Geometry check sheet. Reference: drawing and pictorial views, mm from the part's lowest x, y, z. A direction names the side the tool comes from. Round coordinates to 2 decimals unless told otherwise and drop trailing zeros. Write each loop counter-clockwise with the first axis right and the second up, starting at its lowest first coordinate (ties: lowest second). Pieces come first, ordered by that corner, then holes. Notation, with made-up numbers: M 10,56 L 60,56 A22 cw 60,69 Z; hole C -29.5,51.25 d10. An arc over 180 degrees is marked long. Put each result on its own line as item: value. Start each with the question number.
(1) Section check C-C on y = 46. Record the cut outline in (x, z) (1 decimal).
(2) Gauge pin test, flat ends, axial feed: pin 1 (5 mm diameter, centred on x = 51.5, z = 8, fed in from -Y); pin 2 (12 mm diameter, centred on x = 24, z = 3.5, fed in from +Y); pin 3 (8 mm diameter, centred on x = 60.5, z = 18, fed in from +Y); pin 4 (2.5 mm diameter, centred on x = 20.05, y = 46, fed in from -Z). Record the tip position at first contact, or that the pin passes through.
(3) Section check D-D on x = 26.5. Record the cut outline in (y, z) (1 decimal), then the cut area to 3 significant figures.
(4) Material ranges on probe 1 along Y at (x, z) = (36.5, 1.15); probe 2 along Y at (x, z) = (36, 6) (1 decimal); probe 3 along Y at (x, z) = (37.5, 27.5) (1 decimal), recorded low to high.
(5) Section check B-B on z = 18.5. Record the cut outline in (x, y) (1 decimal).
(6) Mould release check, pull along Y, two halves, no side actions. Record for the marked faces 1, 2 and 3: pulls with the +Y half, pulls with the -Y half, needs draft (parallel to the pull), parting line crosses it, or undercut.
(7) Tool access check on the marked faces 4, 5, 6, 7 and 8. Record the directions out of +Z, -Z, +X, -X, +Y, -Y that give a thin tool (end or side, any length) a straight path to the whole face; none if there is none.
(8) Section check A-A on x = 36.5. Count the separate pieces of the cut face and the enclosed holes in it, then the cut area to 3 significant figures.
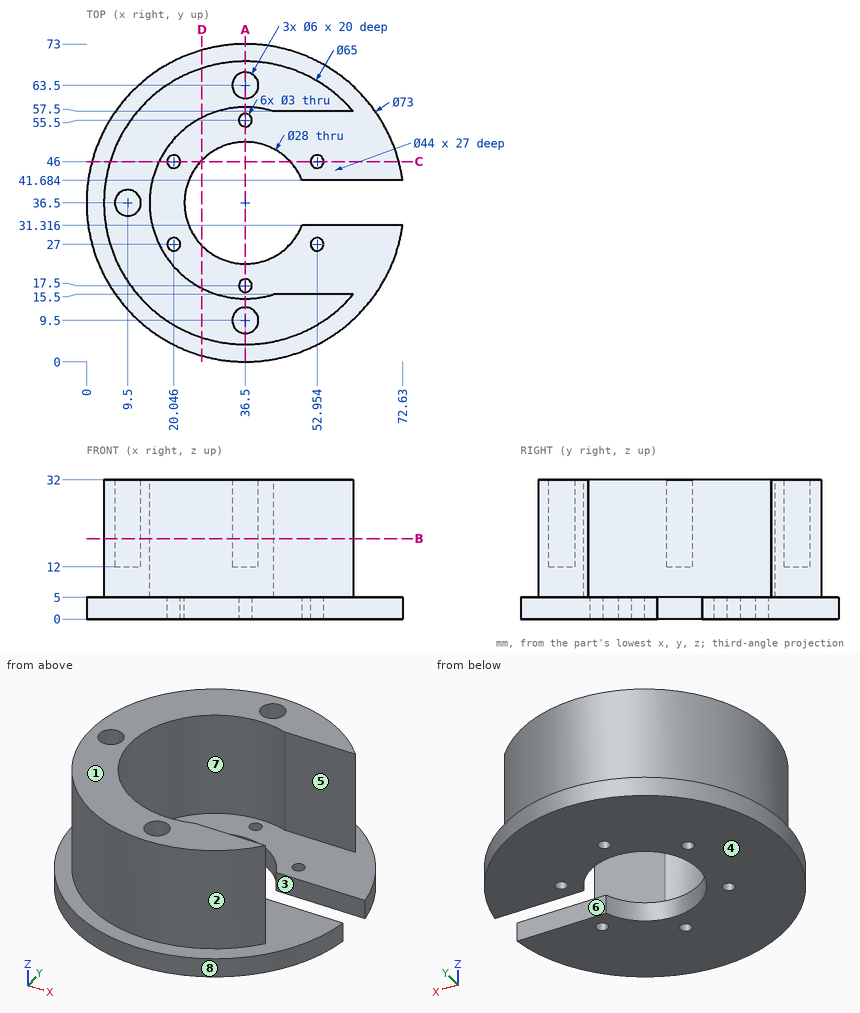
Answers follow:
1. outline: M 1.3,0 L 18.5,0 L 18.5,5 L 16.7,5 L 16.7,32 L 5.4,32 L 5.4,5 L 1.3,5 Z; M 21.5,0 L 26.2,0 L 26.2,5 L 21.5,5 Z; M 46.8,0 L 51.5,0 L 51.5,5 L 46.8,5 Z; M 54.5,0 L 71.7,0 L 71.7,5 L 54.5,5 Z
2. pin 1: stops at y = 6.5
2. pin 2: stops at y = 72.42
2. pin 3: stops at y = 62.12
2. pin 4: passes through
3. outline: M 1.4,0 L 26.7,0 L 26.7,5 L 16.9,5 L 16.9,32 L 5.6,32 L 5.6,5 L 1.4,5 Z; M 46.3,0 L 71.6,0 L 71.6,5 L 67.4,5 L 67.4,32 L 56.1,32 L 56.1,5 L 46.3,5 Z
3. area: 865 mm^2
4. probe 1: y = 0 to 16, 19 to 22.5, 50.5 to 54, 57 to 73
4. probe 2: y = 4 to 14.5, 58.5 to 69
4. probe 3: y = 4 to 6.7, 12.3 to 14.5, 58.5 to 60.7, 66.3 to 69
5. outline: M 43.1,15.5 A22 cw long 43.1,57.5 L 61.3,57.5 A32.5 ccw long 61.3,15.5 Z; hole C 9.5,36.5 d6; hole C 36.5,9.5 d6; hole C 36.5,63.5 d6
6. face 1: needs draft
6. face 2: parting line crosses it
6. face 3: undercut
7. face 4: -Z, +X, -X, +Y, -Y
7. face 5: +Z, +X
7. face 6: +Z, -Z, +X
7. face 7: +Z
7. face 8: +Z, -Z
8. separate pieces: 4
8. enclosed holes: 0
8. area: 522 mm^2
